Input: dimensioned drawing with shaded views. Units: mm. Origin: part minimum x, y, z. A direction names the side the tool comes from. Round coordinates to 2 decimals unless told otherwise and drop trailing zeros. Write each loop counter-clockwise with the first axis right and the second up, starting at its lowest first coordinate (ties: lowest second). Pieces come first, ordered by that corner, then holes. Notation, with made-up numbers: (18, 52.25) - (54, 52.25) arc R17 cw to (54, 67.25) - close; hole circle Ø7 at (37.25, 56.5). An arc over 180 degrees is marked (long way). Write item = value, one per line. Start each with the question number.
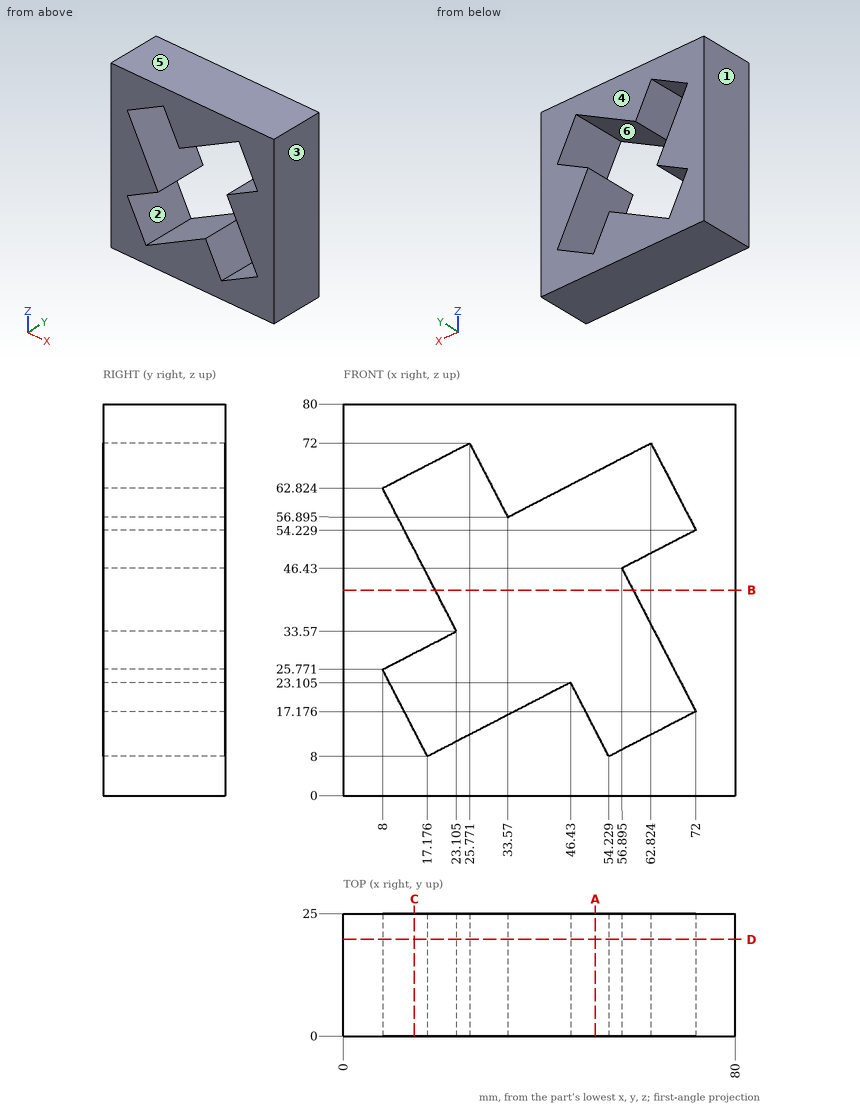
(1) Reachability of the marked faces 5 and 6 from +Z, -Z, +X, -X, +Y, -Y: full face, straight path, thin tool, end or side. Return the list, or none.
(2) Pull-direction query (X, two-part tool) for the marked faces 1, 2, 3 and 4; classes: +X half, -X half, draft (parallel to the pull), parting line (faces both ways), or undercut.
(3) Contact query for a flat-ended pin moving along its axis: P1, Ø10, axis at x = 48, z = 46.5, coming from the +Y side. Output: stop coordinate, or through.
(4) Section D-D (y = 19.75). Return the cut outline in (x, z) (1 decimal), plus the area to 3 significant figures.
(5) Section B-B (z = 42). Return the cut outline in (x, y), plus the area to 3 significant figures.
(6) Ray query, L1, parallel to X at y = 19.25, z = 60 (1 decimal); L2, parallel to Z at x = 14.5, y = 4 (1 decimal); L3, parallel to X at y = 3.25, z = 16.5 (1 decimal). Return the intervals inside material, ascending. Write a range as from..to.
(7) Section A-A (x = 51.5). Return the cut outline in (y, z) (1 decimal).
(8) Section C-C (x = 14.5). Return the cut outline in (y, z) (1 decimal).
Solution:
q1.face_5 = +Z, +X, -X, +Y, -Y
q1.face_6 = +Y, -Y
q2.face_1 = -X half
q2.face_2 = undercut
q2.face_3 = +X half
q2.face_4 = draft
q3.P1 = through
q4.outline = (0, 0) - (80, 0) - (80, 80) - (0, 80) - close; hole (8, 25.8) - (17.2, 8) - (46.4, 23.1) - (54.2, 8) - (72, 17.2) - (56.9, 46.4) - (72, 54.2) - (62.8, 72) - (33.6, 56.9) - (25.8, 72) - (8, 62.8) - (23.1, 33.6) - close
q4.area = 3,750 mm^2
q5.outline = (0, 0) - (18.75, 0) - (18.75, 25) - (0, 25) - close; (59.18, 0) - (80, 0) - (80, 25) - (59.18, 25) - close
q5.area = 989 mm^2
q6.L1 = 0..9.5, 32..39.6, 69..80
q6.L2 = 0..13.2, 29.1..50.2, 66.2..80
q6.L3 = 0..12.8, 33.6..49.8, 70.7..80
q7.outline = (0, 0) - (25, 0) - (25, 13.3) - (0, 13.3) - close; (0, 66.2) - (25, 66.2) - (25, 80) - (0, 80) - close
q8.outline = (0, 0) - (25, 0) - (25, 13.2) - (0, 13.2) - close; (0, 29.1) - (25, 29.1) - (25, 50.2) - (0, 50.2) - close; (0, 66.2) - (25, 66.2) - (25, 80) - (0, 80) - close
